Autodesk Inventor part; units mm, degrees
ref_plane "YZ Plane" through (0, 0, 0) normal (1, 0, 0) x (0, 1, 0)
ref_plane "XZ Plane" through (0, 0, 0) normal (0, 1, 0) x (-1, 0, 0)
ref_plane "XY Plane" through (0, 0, 0) normal (0, 0, 1) x (1, 0, 0)
sketch "Sketch1" plane through (0, 0, 0) normal (0, 1, 0) x (-1, 0, 0)
  circle A0 centre (0, 0) radius 55
  dimension "d0" = 110
extrude "Extrusion1" add sketch "Sketch1" against normal blind 10
sketch "Sketch2" plane through (0, 0, 0) normal (0, 1, 0) x (1, 0, 0)
  circle A0 centre (0, 0) radius 55
  line L0 (-7.5, 54) -> (7.5, 54)
  line L1 (7.5, 54) -> (7.5, 62.0467)
  line L2 (7.5, 62.0467) -> (-7.5, 62.0467)
  line L3 (-7.5, 62.0467) -> (-7.5, 54)
  point P0 (0, 54)
  point P1 (7.5, 54.4862)
  point P2 (-7.5, 54.4862)
  point P3 (0, 62.0467)
  dimension "d3" = 15
  dimension "d4" = 8.0467
  dimension "d21" = 62.0467
extrude "Extrusion2" add sketch "Sketch2" along normal blind 5 and the other way blind 10 contours L1 L0 L3 A0 | A0 L3 L2 L1 picked at (0.8356, 54.3143)
sketch "Sketch3" plane through (-7.5, 0, -54) normal (0, 0, 1) x (1, 0, 0)
  line L0 (15, 0) -> (0, 0)
  line L1 (0, 5) -> (15, 5)
  line L2 (0, 5) -> (15, 5)
  line L3 (0, 5) -> (0, 8.9533)
  line L4 (15, 5) -> (15, 8.9533)
  arc A0 (15, 8.9533) -> (0, 8.9533) centre (7.5, 17) ccw
  line L5 (0, 5) -> (15, 5)
  point P0 (7.5, 0)
  point P1 (7.5, 0)
  point P2 (7.5, 5)
  point P3 (7.5, 5)
  dimension "d27" = 22
  dimension "d28" = 12
  dimension "d29" = 15
extrude "Extrusion3" add sketch "Sketch3" against normal up to surface (8.0467 mm away)
pattern_circular "Circular Pattern1" count 3 over 360 about axis through (0, 0, 0) along (0, -1, 0) of "Extrusion2", "Extrusion3"
sketch "Sketch5" plane through (-7.5, 0, -54) normal (0, 0, 1) x (1, 0, 0)
  arc A0 (15, 8.9533) -> (0, 8.9533) centre (7.5, 17) ccw
  circle A1 centre (7.5, 17) radius 2.4
  point P0 (7.5, 0)
  dimension "d30" = 4.8
extrude "Extrusion5" add sketch "Sketch5" against normal blind 24
pattern_circular "Circular Pattern3" count 3 over 360 about axis through (0, 0, 0) along (0, -1, 0) of "Extrusion5"
sketch "Sketch6" plane through (-50.5154, 0, 20.5048) normal (0.866, 0, -0.5) x (-0.5, 0, -0.866)
  arc A0 (0, 8.9533) -> (-15, 8.9533) centre (-7.5, 17) ccw
  arc A1 (0, 8.9533) -> (-15, 8.9533) centre (-7.5, 17) ccw
  line L0 (-4.3246, 17) -> (-5.9123, 14.25)
  line L1 (-5.9123, 14.25) -> (-9.0877, 14.25)
  line L2 (-9.0877, 14.25) -> (-10.6754, 17)
  line L3 (-10.6754, 17) -> (-9.0877, 19.75)
  line L4 (-9.0877, 19.75) -> (-5.9123, 19.75)
  line L5 (-5.9123, 19.75) -> (-4.3246, 17)
  point P0 (-7.5, 0)
  dimension "d36" = 5.5
extrude "Extrusion6" cut sketch "Sketch6" against normal blind 3
sketch "Sketch7" plane through (-53.1134, 0, 22.0048) normal (0.866, 0, -0.5) x (-0.5, 0, -0.866)
  circle A0 centre (-7.5, 17) radius 1.6
  line L0 (-9.0877, 19.75) -> (-5.9123, 19.75)
  line L1 (-10.6754, 17) -> (-9.0877, 19.75)
  line L2 (-9.0877, 14.25) -> (-10.6754, 17)
  line L3 (-5.9123, 14.25) -> (-9.0877, 14.25)
  line L4 (-4.3246, 17) -> (-5.9123, 14.25)
  line L5 (-5.9123, 19.75) -> (-4.3246, 17)
  point P0 (-7.5, 0)
  point P1 (-7.5, 14.25)
  dimension "d39" = 3.2
extrude "Extrusion7" cut sketch "Sketch7" against normal through all contours A0
pattern_circular "Circular Pattern4" count 3 over 360 about axis through (0, 0, 0) along (0, -1, 0) of "Extrusion6", "Extrusion7"
properties part number "mobile_platform"
Geometry check sheet. Reference: the model listing, model coordinates, mm. A direction names the side the tool comes from. Give positions to 0.01 mm unless a question says otherwise; leave off trailing zeros. Order: outer loops, then holes, each group sorted by start corner. A loop starts at its lowest first (then second) coordinate and runs counter-clockwise, first axis right, second up.
1) Cross-section at C-C (y = 23). Record the boundary of the cut face in (x, z), then the cut area to 3 significant figures.
Results are:
outline: (-58.34, 23.04) - (-51.38, 19.02) - (-42.16, 34.98) - (-49.12, 39.01) - close; (-9.22, -62.05) - (9.22, -62.05) - (9.22, -54) - (-9.22, -54) - close; (42.16, 34.98) - (51.38, 19.02) - (58.34, 23.04) - (49.12, 39.01) - close
area: 445 mm2
2) Cross-section at D-D (x = 34). Record the boundary of the cut face in (y, z).
Results are:
outline: (-10, -43.23) - (0, -43.23) - (0, 43.23) - (-10, 43.23) - close
3) Tool access check on faces 1 (the flat face through (-50.049, 18.261, 27.317)), 2 (the flat face through (0, 14, -54)), 3 (the flat face through (0, 19.75, -55)). Record the directions out of +Z, -Z, +X, -X, +Y, -Y that give a thin tool (end or side, any length) a straight path to the whole face; none if there is none.
Results are:
face 1: none
face 2: +Z, +X, -X, +Y
face 3: +Z
4) Cross-section at A-A (x = 0). Record the boundary of the cut face in (y, z), then the cut area to 3 significant figures.
Results are:
outline: (-10, -62.05) - (14.6, -62.05) - (14.6, -78) - (15.4, -78) - (15.4, -57) - (14.25, -57) - (14.25, -54) - (0, -54) - (0, 55) - (-10, 55) - close; (18.6, -78) - (19.4, -78) - (19.4, -62.05) - (28, -62.05) - (28, -54) - (19.75, -54) - (19.75, -57) - (18.6, -57) - close
area: 1,390 mm2
5) Gauge pin test, flat ends, axial feed: pin 1 (1 mm diameter, centred on x = 53, z = 11.5, fed in from +Y); pin 2 (4 mm diameter, centred on y = -0.5, z = -57.5, fed in from -X); pin 3 (1.5 mm diameter, centred on x = -1, z = -55.5, fed in from +Y); pin 4 (1.6 mm diameter, centred on x = -0.5, y = 17.5, fed in from +Z). Record the tip position at first contact, or that the pin passes through.
Results are:
pin 1: stops at y = 0
pin 2: stops at x = -7.5
pin 3: stops at y = 28
pin 4: passes through
6) Material ranges on probe 1 along Y at (x, z) = (-2, -39); probe 2 along Z at (x, y) = (54.5, 22); probe 3 along Z at (x, y) = (-53.5, 21.5), recorded low to high.
Results are:
probe 1: y = -10 to 0
probe 2: z = 20.15 to 29.7
probe 3: z = 19.3 to 31.43
7) Cross-section at B-B (y = 5.5). Record the boundary of the cut face in (x, z).
Results are:
outline: (-57.48, 24.53) - (-50.52, 20.5) - (-43.02, 33.5) - (-49.98, 37.52) - close; (-7.5, -62.05) - (7.5, -62.05) - (7.5, -54) - (-7.5, -54) - close; (43.02, 33.5) - (50.52, 20.5) - (57.48, 24.53) - (49.98, 37.52) - close
8) Draft check along X on faces 4 (the flat face through (53.95, -0.66, 22.49)), 5 (the flat face through (-53.95, -0.66, 22.49)), 6 (the flat face through (2, 17, -78)), 7 (the flat face through (-48, 19.75, 28)). Enter one of: released by +X, released by -X, zero draft, split by the parting line, or undercut.
Results are:
face 4: released by +X
face 5: released by -X
face 6: zero draft
face 7: undercut
